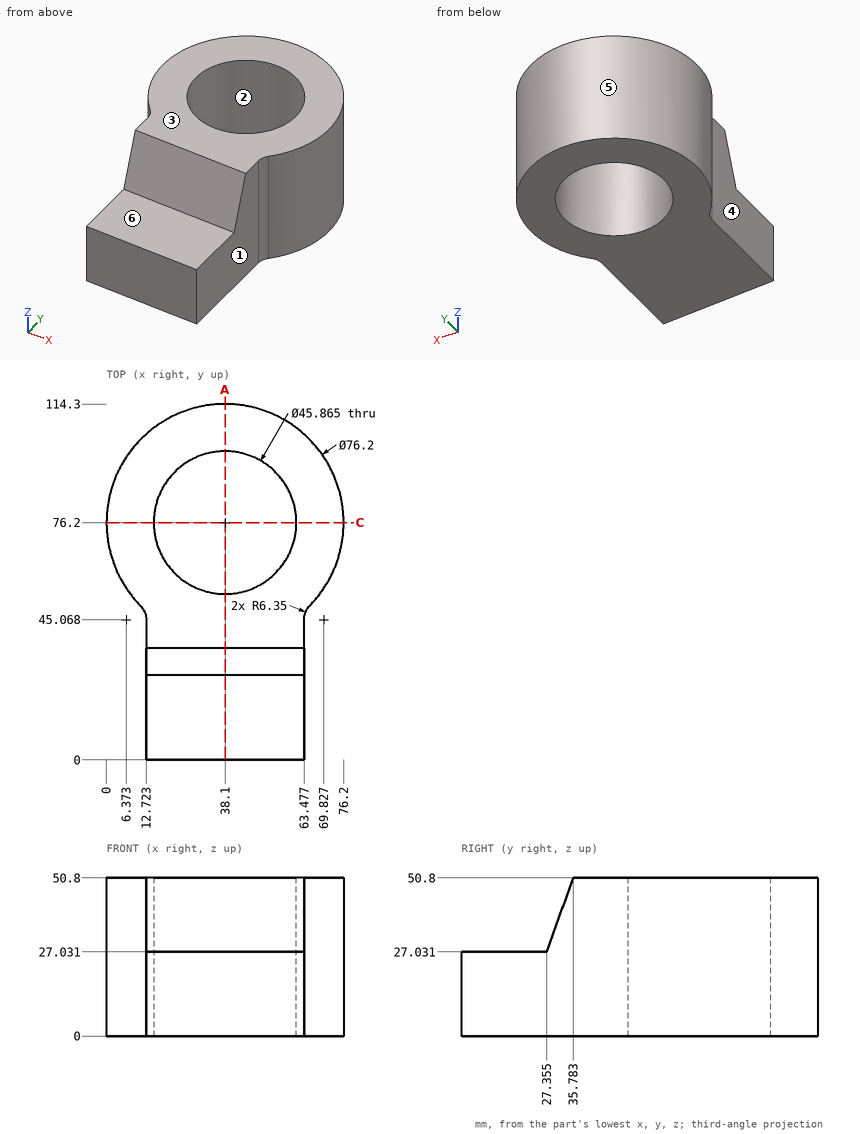
Answer from the drawing. Dimensions are ordinates in mm from the lowest x, y and z of the part. A direction names the side the tool comes from. Give positions to 0.01 mm unless a question says otherwise; leave off trailing zeros. Order: outer loops, then holes, each group sorted by start corner. A loop starts at its lowest first (then second) coordinate and runs counter-clockwise, first axis right, second up. Notation, with made-up numbers: (19.5, -11) - (33.5, -11) arc R5 cw to (33.5, -4) - close; hole circle Ø11 at (-36.5, 67). An arc over 180 degrees is marked (long way). Use one line per item in the form item = value.
1) Find section A-A on x = 38.1. Determine the outline of the cut face in (y, z) (1 decimal).
Verdict:
outline = (0, 0) - (53.3, 0) - (53.3, 50.8) - (35.8, 50.8) - (27.4, 27) - (0, 27) - close; (99.1, 0) - (114.3, 0) - (114.3, 50.8) - (99.1, 50.8) - close
2) Find section C-C on y = 76.2. Determine the outline of the cut face in (x, z), and give its area (3 significant figures).
Verdict:
outline = (0, 0) - (15.17, 0) - (15.17, 50.8) - (0, 50.8) - close; (61.03, 0) - (76.2, 0) - (76.2, 50.8) - (61.03, 50.8) - close
area = 1,540 mm^2
3) For the marked faces 5 and 6, determine the directions among +Z, -Z, +X, -X, +Y, -Y from which every point of the face is accessible in a straight line to the end or side of a thin tool.
Verdict:
face_5 = +Z, -Z
face_6 = +Z, +X, -X, -Y
4) Each of these flat-tipped pins is pushed along its axis until it touches: pin 1 (3 mm diameter, centred on y = 23, z = 27, fed in from +X); pin 2 (1.5 mm diameter, centred on y = 55, z = 13, fed in from -X); pin 3 (10 mm diameter, centred on y = 42.5, z = 13.5, fed in from +X). Where does it stop, or does it pass through?
Verdict:
pin_1 = 63.48
pin_2 = 5.95
pin_3 = 63.96
5) Consider probe 1 along Y at (x, z) = (38.1, 22); probe 2 along X at (y, z) = (76, 23); probe 3 along Z at (x, y) = (26.5, 6). Determine where each line is inside the solid, lowest interval first. Write a range as [from, to].
Verdict:
probe_1 = [0, 53.27], [99.13, 114.3]
probe_2 = [0, 15.17], [61.03, 76.2]
probe_3 = [0, 27.03]
6) The mould has two halves that part along X. Classify the marked faces 1, 2, 3 and 4: released by +X, released by -X, zero draft, split by the parting line, or undercut.
Verdict:
face_1 = released by +X
face_2 = undercut
face_3 = zero draft
face_4 = released by -X
